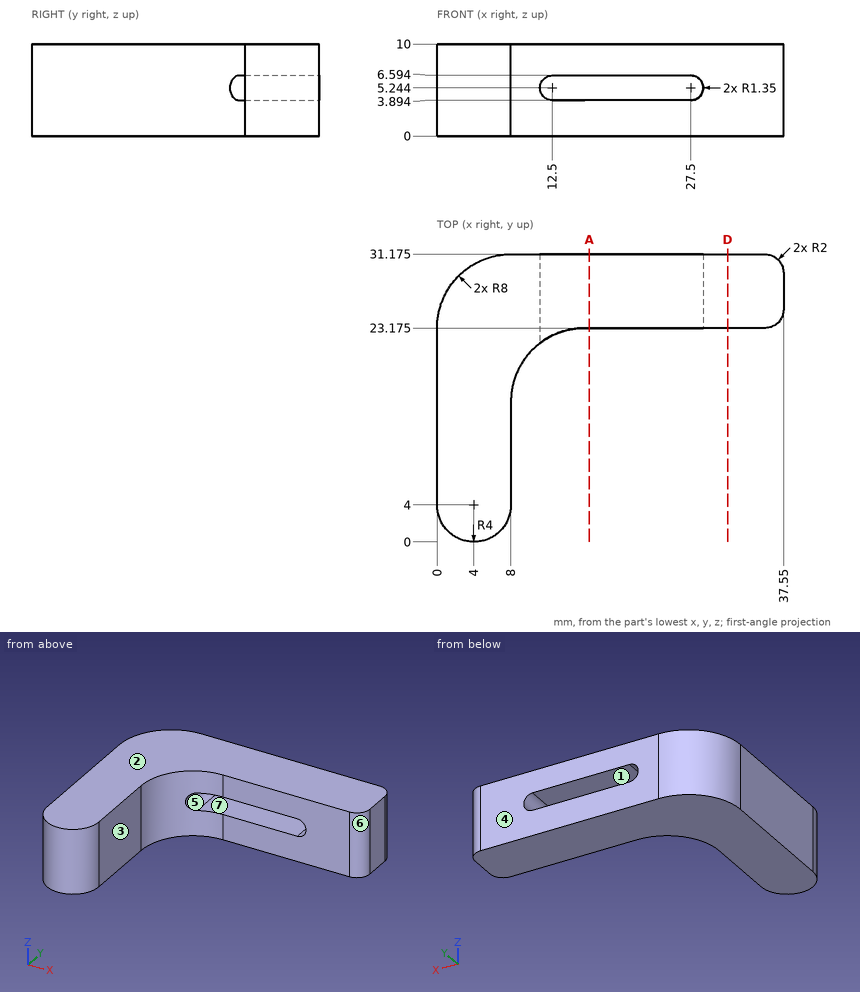
Answer from the drawing. Dimensions are ordinates in mm from the lowest x, y and z of the part. A direction names the side the tool comes from. Coordinates: 2 decimals unless noted, no trailing zeros. Loops run counter-clockwise (first coordinate to the right, second up) from the corner with the lowest first, then second, coordinate; pieces in that order, holes last. Notation, with made-up numbers: (46.5, 68.25) - (80.5, 68.25) arc R24 ccw to (80.5, 88.25) - close; hole circle Ø6 at (46.25, 55). An arc over 180 degrees is marked (long way). Answer in a Markdown table with one row per item.
1. Find section A-A, the plane x = 16.5. Write down the section's boundary in (y, z) (1 decimal).
Conclusion:
| item | result |
|---|---|
| outline | (23.2, 0) - (31.2, 0) - (31.2, 3.9) - (23.2, 3.9) - close; (23.2, 6.6) - (31.2, 6.6) - (31.2, 10) - (23.2, 10) - close |
2. Find section D-D, the plane x = 31.5. Write down the section's boundary in (y, z) (1 decimal).
Conclusion:
| item | result |
|---|---|
| outline | (23.2, 0) - (31.2, 0) - (31.2, 10) - (23.2, 10) - close |
3. Given pin 1 (1 mm diameter, centred on x = 16.5, z = 6, fed in from +Y); pin 2 (5 mm diameter, centred on y = 10.5, z = 2.5, fed in from +X); pin 3 (2 mm diameter, centred on x = 7, z = 5, fed in from +Y) (3 decimals); pin 4 (3 mm diameter, centred on x = 21, z = 3.5, fed in from -Y) (3 decimals), each flat-ended and moving along its own axis, determine where each tip first touches the part or whether it passes through.
Conclusion:
| item | result |
|---|---|
| pin 1 | passes through |
| pin 2 | stops at x = 8 |
| pin 3 | stops at y = 31.175 |
| pin 4 | stops at y = 23.175 |
4. Straight lines are drawn through the part: line 1 (Z direction, x = 19, y = 29.5); line 2 (X direction, y = 14, z = 2.75); line 3 (Y direction, x = 20, z = 1.5) (1 decimal). For each, find the intervals that lie inside material, in ascending order.
Conclusion:
| item | result |
|---|---|
| line 1 | z = 0 to 3.89, 6.59 to 10 |
| line 2 | x = 0 to 8 |
| line 3 | y = 23.2 to 31.2 |
5. Determine the mould class of the marked faces 4, 5, 6 and 7 for opening direction X: +X half, -X half, draft (parallel to the pull), parting line (faces both ways), or undercut.
Conclusion:
| item | result |
|---|---|
| face 4 | draft |
| face 5 | undercut |
| face 6 | +X half |
| face 7 | undercut |
6. Which of the six approach directions +Z, -Z, +X, -X, +Y, -Y give full straight-line access (tool end or side, diameter ignored) to the marked faces 1, 2 and 3?
Conclusion:
| item | result |
|---|---|
| face 1 | +Y, -Y |
| face 2 | +Z, +X, -X, +Y, -Y |
| face 3 | +Z, -Z, +X, -Y |
